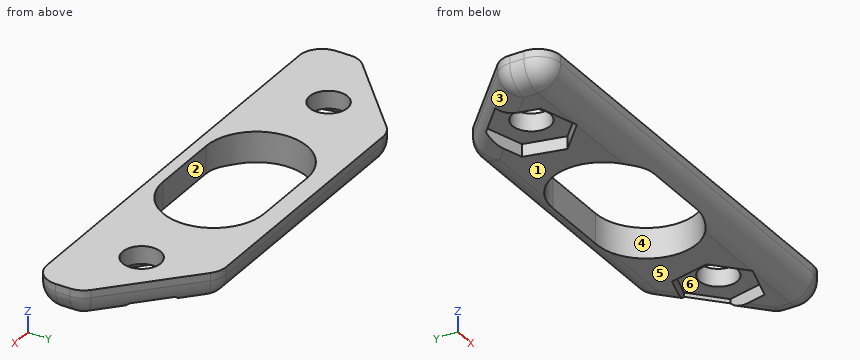
from build123d import *

# Parameters (mm, degrees)
F0_R         = 1.5
F1_DEPTH     = 2.4
F2_DEPTH     = 1
F3_T1_DEPTH  = 1.1190522621
F3_T3_DEPTH  = 32.4
F3_T5_DEPTH  = 20.138628613
F3_T7_DEPTH  = 2.365520331
F3_T9_DEPTH  = 8.3614446785
F3_T11_DEPTH = 8.3614446785
F3_T13_DEPTH = 5.1
F3_T15_DEPTH = 2.5639483811
F3_T20_DEPTH = 1.8
F3_S25_W     = 1.8
F3_S25_H     = 1.8
F3_T26_DEPTH = 1.8
F3_S31_W     = 1.8
F3_S31_H     = 1.8
F3_T32_DEPTH = 1.8
F3_T38_DEPTH = 1.8
F3_T44_DEPTH = 1.8
F3_T50_DEPTH = 1.8


# Not quite as in the source:
# - a fillet or chamfer that OpenCascade refuses, or shapes differently, is made with other operations: its cross-section is extruded or revolved along the edge and cut away or added


with BuildPart() as f1:
    # F0 (on Top) → F1 (new body)
    with BuildSketch(Plane.XY):
        Polygon((-18, -1.2002319389), (-18, -4.9048635534), (18, -4.9048635534), (18, -1.2002319389), (10.7755224389, 5.5), (-10.7755224389, 5.5), align=None)
        Polygon((-9.6294171928, 2.1985610038), (-8.9106989153, -0.9537044309), (-11.2812817225, -3.1522654347), (-14.3705828072, -2.1985610038), (-15.0893010847, 0.9537044309), (-12.7187182775, 3.1522654347), align=None, mode=Mode.SUBTRACT)
        with BuildLine():
            ThreePointArc((-2.75, -4), (-6.75, 0), (-2.75, 4))
            Line((-2.75, 4), (2.75, 4))
            ThreePointArc((2.75, 4), (6.75, 0), (2.75, -4))
            Line((2.75, -4), (-2.75, -4))
        make_face(mode=Mode.SUBTRACT)
        Polygon((9.6294171928, 2.1985610038), (12.7187182775, 3.1522654347), (15.0893010847, 0.9537044309), (14.3705828072, -2.1985610038), (11.2812817225, -3.1522654347), (8.9106989153, -0.9537044309), align=None, mode=Mode.SUBTRACT)
        Polygon((-11.2812817225, -3.1522654347), (-8.9106989153, -0.9537044309), (-9.6294171928, 2.1985610038), (-12.7187182775, 3.1522654347), (-15.0893010847, 0.9537044309), (-14.3705828072, -2.1985610038), align=None)
        with Locations((-12, 0)):
            Circle(F0_R, mode=Mode.SUBTRACT)
        Polygon((15.0893010847, 0.9537044309), (12.7187182775, 3.1522654347), (9.6294171928, 2.1985610038), (8.9106989153, -0.9537044309), (11.2812817225, -3.1522654347), (14.3705828072, -2.1985610038), align=None)
        with Locations((12, 0)):
            Circle(F0_R, mode=Mode.SUBTRACT)
    extrude(amount=F1_DEPTH)

    # F0 (on Top) → F2 (cut)
    with BuildSketch(Plane.XY):
        Polygon((15.0893010847, 0.9537044309), (12.7187182775, 3.1522654347), (9.6294171928, 2.1985610038), (8.9106989153, -0.9537044309), (11.2812817225, -3.1522654347), (14.3705828072, -2.1985610038), align=None)
        with Locations((12, 0)):
            Circle(F0_R, mode=Mode.SUBTRACT)
        Polygon((-11.2812817225, -3.1522654347), (-8.9106989153, -0.9537044309), (-9.6294171928, 2.1985610038), (-12.7187182775, 3.1522654347), (-15.0893010847, 0.9537044309), (-14.3705828072, -2.1985610038), align=None)
        with Locations((-12, 0)):
            Circle(F0_R, mode=Mode.SUBTRACT)
    extrude(amount=F2_DEPTH, mode=Mode.SUBTRACT)

    # F3: fillet of radius 1.8 on 12 edges, made by hand

    # F3_s2 → F3_t1 (cut)
    with BuildSketch(Plane.XZ.offset(1.9858112913)):
        with BuildLine():
            ThreePointArc((-18, 1.8), (-17.4727922061, 0.5272077939), (-16.2, 0))
            Line((-16.2, 0), (-18, 0))
            Line((-18, 0), (-18, 1.8))
        make_face()
        with BuildLine():
            ThreePointArc((16.2, 0), (17.4727922061, 0.5272077939), (18, 1.8))
            Line((18, 1.8), (18, 0))
            Line((18, 0), (16.2, 0))
        make_face()
    extrude(amount=F3_T1_DEPTH, mode=Mode.SUBTRACT)

    # F3_s4 → F3_t3 (cut)
    with BuildSketch(Plane.YZ.offset(-16.2)):
        with BuildLine():
            ThreePointArc((-4.9048635534, 1.8), (-4.3776557595, 0.5272077939), (-3.1048635534, 0))
            Line((-3.1048635534, 0), (-4.9048635534, 0))
            Line((-4.9048635534, 0), (-4.9048635534, 1.8))
        make_face()
    extrude(amount=F3_T3_DEPTH, mode=Mode.SUBTRACT)

    # F3_s6 → F3_t5 (cut)
    with BuildSketch(Plane.YZ.offset(-10.0693143065)):
        with BuildLine():
            ThreePointArc((3.7, 0), (4.9727922061, 0.5272077939), (5.5, 1.8))
            Line((5.5, 1.8), (5.5, 0))
            Line((5.5, 0), (3.7, 0))
        make_face()
    extrude(amount=F3_T5_DEPTH, mode=Mode.SUBTRACT)

    # F3_s8 → F3_t7 (cut)
    with BuildSketch(Plane.XY.offset(1.8)):
        with BuildLine():
            ThreePointArc((10.0693143065, 5.5), (10.7267347006, 5.3756486581), (11.2933205301, 5.0197760282))
            Line((11.2933205301, 5.0197760282), (10.7755224389, 5.5))
            Line((10.7755224389, 5.5), (10.0693143065, 5.5))
        make_face()
        with BuildLine():
            ThreePointArc((-11.2933205301, 5.0197760282), (-10.7267347006, 5.3756486581), (-10.0693143065, 5.5))
            Line((-10.0693143065, 5.5), (-10.7755224389, 5.5))
            Line((-10.7755224389, 5.5), (-11.2933205301, 5.0197760282))
        make_face()
    extrude(amount=F3_T7_DEPTH, mode=Mode.SUBTRACT)

    # F3_s10 → F3_t9 (cut)
    with BuildSketch(Plane(origin=(-3.5684530391, -3.3095075488, 0), x_dir=(0, 0, 1), z_dir=(-0.7332089046, -0.6800034575, 0))):
        with BuildLine():
            ThreePointArc((1.8, 11.3600414903), (0.5272077939, 10.8328336964), (0, 9.5600414903))
            Line((0, 9.5600414903), (0, 11.3600414903))
            Line((0, 11.3600414903), (1.8, 11.3600414903))
        make_face()
    extrude(amount=F3_T9_DEPTH, mode=Mode.SUBTRACT)

    # F3_s12 → F3_t11 (cut)
    with BuildSketch(Plane(origin=(9.6991387326, -8.9953188401, 0), x_dir=(0, 0, 1), z_dir=(-0.7332089046, 0.6800034575, 0))):
        with BuildLine():
            ThreePointArc((0, 9.5600414903), (0.5272077939, 10.8328336964), (1.8, 11.3600414903))
            Line((1.8, 11.3600414903), (0, 11.3600414903))
            Line((0, 11.3600414903), (0, 9.5600414903))
        make_face()
    extrude(amount=F3_T11_DEPTH, mode=Mode.SUBTRACT)

    # F3_s14 → F3_t13 (cut)
    with BuildSketch(Plane.XY.offset(1.8)):
        with BuildLine():
            ThreePointArc((-18, -3.1048635534), (-17.4727922061, -4.3776557595), (-16.2, -4.9048635534))
            Line((-16.2, -4.9048635534), (-18, -4.9048635534))
            Line((-18, -4.9048635534), (-18, -3.1048635534))
        make_face()
        with BuildLine():
            ThreePointArc((16.2, -4.9048635534), (17.4727922061, -4.3776557595), (18, -3.1048635534))
            Line((18, -3.1048635534), (18, -4.9048635534))
            Line((18, -4.9048635534), (16.2, -4.9048635534))
        make_face()
    extrude(amount=F3_T13_DEPTH, mode=Mode.SUBTRACT)

    # F3_s16 → F3_t15 (cut)
    with BuildSketch(Plane.XY.offset(1.8)):
        with BuildLine():
            ThreePointArc((-18, -1.9858112913), (-17.8497289478, -1.265815181), (-17.4240062235, -0.666035263))
            Line((-17.4240062235, -0.666035263), (-18, -1.2002319389))
            Line((-18, -1.2002319389), (-18, -1.9858112913))
        make_face()
        with BuildLine():
            ThreePointArc((18, -1.9858112913), (17.8497289478, -1.265815181), (17.4240062235, -0.666035263))
            Line((17.4240062235, -0.666035263), (18, -1.2002319389))
            Line((18, -1.2002319389), (18, -1.9858112913))
        make_face()
    extrude(amount=F3_T15_DEPTH, mode=Mode.SUBTRACT)


with BuildPart() as f3_tool18:
    # F3_s19 → F3_t20 (new body)
    with BuildSketch(Plane.XY.offset(1.8)):
        Polygon((-16.2, -1.9858112913), (-18, -1.9858112913), (-18, -1.2002319389), (-17.4240062235, -0.666035263), align=None)
    extrude(amount=-F3_T20_DEPTH)

    # F3_s21 → F3_t22 (revolve, cut)
    with BuildSketch(Plane(origin=(-16.2, -1.9858112913, 1.8), x_dir=(0.9165160821, -0.399997839, 0), z_dir=(0.399997839, 0.9165160821, 0))):
        with BuildLine():
            ThreePointArc((0, -1.8), (1.8, 0), (0, 1.8))
            Line((0, 1.8), (0, -1.8))
        make_face()
    revolve(axis=Axis((-16.2, -1.9858112913, 1.8), (0, 0, -1)), mode=Mode.SUBTRACT)


with BuildPart() as f1_1:
    add(f1.part)

    # F3_t17: cut F3_tool18
    add(f3_tool18.part, mode=Mode.SUBTRACT)


with BuildPart() as f3_tool24:
    # F3_s25 → F3_t26 (new body)
    with BuildSketch(Plane.YZ.offset(-16.2)):
        with Locations((-4.0048635534, 0.9)):
            Rectangle(F3_S25_W, F3_S25_H)
    extrude(amount=-F3_T26_DEPTH)

    # F3_s27 → F3_t28 (revolve, cut)
    with BuildSketch(Plane(origin=(-16.2, -3.1048635534, 1.8), x_dir=(0, 0.7071067812, 0.7071067812), z_dir=(0, -0.7071067812, 0.7071067812))):
        with BuildLine():
            ThreePointArc((0, -1.8), (1.8, 0), (0, 1.8))
            Line((0, 1.8), (0, -1.8))
        make_face()
    revolve(axis=Axis((-16.2, -3.1048635534, 1.8), (-1, 0, 0)), mode=Mode.SUBTRACT)


with BuildPart() as f1_2:
    add(f1_1.part)

    # F3_t23: cut F3_tool24
    add(f3_tool24.part, mode=Mode.SUBTRACT)


with BuildPart() as f3_tool30:
    # F3_s31 → F3_t32 (new body)
    with BuildSketch(Plane.XZ.offset(3.1048635534)):
        with Locations((17.1, 0.9)):
            Rectangle(F3_S31_W, F3_S31_H)
    extrude(amount=F3_T32_DEPTH)

    # F3_s33 → F3_t34 (revolve, cut)
    with BuildSketch(Plane(origin=(16.2, -3.1048635534, 1.8), x_dir=(-0.7071067812, 0, 0.7071067812), z_dir=(0.7071067812, 0, 0.7071067812))):
        with BuildLine():
            ThreePointArc((0, -1.8), (1.8, 0), (0, 1.8))
            Line((0, 1.8), (0, -1.8))
        make_face()
    revolve(axis=Axis((16.2, -3.1048635534, 1.8), (0, -1, 0)), mode=Mode.SUBTRACT)


with BuildPart() as f1_3:
    add(f1_2.part)

    # F3_t29: cut F3_tool30
    add(f3_tool30.part, mode=Mode.SUBTRACT)


with BuildPart() as f3_tool36:
    # F3_s37 → F3_t38 (new body)
    with BuildSketch(Plane.XY.offset(1.8)):
        Polygon((16.2, -1.9858112913), (18, -1.9858112913), (18, -1.2002319389), (17.4240062235, -0.666035263), align=None)
    extrude(amount=-F3_T38_DEPTH)

    # F3_s39 → F3_t40 (revolve, cut)
    with BuildSketch(Plane(origin=(16.2, -1.9858112913, 1.8), x_dir=(-0.9165160821, -0.399997839, 0), z_dir=(0.399997839, -0.9165160821, 0))):
        with BuildLine():
            ThreePointArc((0, -1.8), (1.8, 0), (0, 1.8))
            Line((0, 1.8), (0, -1.8))
        make_face()
    revolve(axis=Axis((16.2, -1.9858112913, 1.8), (0, 0, -1)), mode=Mode.SUBTRACT)


with BuildPart() as f1_4:
    add(f1_3.part)

    # F3_t35: cut F3_tool36
    add(f3_tool36.part, mode=Mode.SUBTRACT)


with BuildPart() as f3_tool42:
    # F3_s43 → F3_t44 (new body)
    with BuildSketch(Plane.XY.offset(1.8)):
        Polygon((10.0693143065, 3.7), (10.0693143065, 5.5), (10.7755224389, 5.5), (11.2933205301, 5.0197760282), align=None)
    extrude(amount=-F3_T44_DEPTH)

    # F3_s45 → F3_t46 (revolve, cut)
    with BuildSketch(Plane(origin=(10.0693143065, 3.7, 1.8), x_dir=(-0.3652335523, -0.9309159212, 0), z_dir=(0.9309159212, -0.3652335523, 0))):
        with BuildLine():
            ThreePointArc((0, -1.8), (1.8, 0), (0, 1.8))
            Line((0, 1.8), (0, -1.8))
        make_face()
    revolve(axis=Axis((10.0693143065, 3.7, 1.8), (0, 0, -1)), mode=Mode.SUBTRACT)


with BuildPart() as f1_5:
    add(f1_4.part)

    # F3_t41: cut F3_tool42
    add(f3_tool42.part, mode=Mode.SUBTRACT)


with BuildPart() as f3_tool48:
    # F3_s49 → F3_t50 (new body)
    with BuildSketch(Plane.XY.offset(1.8)):
        Polygon((-10.0693143065, 3.7), (-10.0693143065, 5.5), (-10.7755224389, 5.5), (-11.2933205301, 5.0197760282), align=None)
    extrude(amount=-F3_T50_DEPTH)

    # F3_s51 → F3_t52 (revolve, cut)
    with BuildSketch(Plane(origin=(-10.0693143065, 3.7, 1.8), x_dir=(0.3652335523, -0.9309159212, 0), z_dir=(0.9309159212, 0.3652335523, 0))):
        with BuildLine():
            ThreePointArc((0, -1.8), (1.8, 0), (0, 1.8))
            Line((0, 1.8), (0, -1.8))
        make_face()
    revolve(axis=Axis((-10.0693143065, 3.7, 1.8), (0, 0, -1)), mode=Mode.SUBTRACT)


with BuildPart() as f1_6:
    add(f1_5.part)

    # F3_t47: cut F3_tool48
    add(f3_tool48.part, mode=Mode.SUBTRACT)


solid = f1_6.part
Model file for the job. Use its own axes, mm. Face numbers are marked on the shaded views. A direction names the side the tool comes from. Coordinates: 2 decimals unless noted, no trailing zeros. Write each loop counter-clockwise with the first axis right and the second up, starting at its lowest first coordinate (ties: lowest second). Pieces come first, ordered by that corner, then holes. Notation, with made-up numbers: (-28.5, 25) - (-22.5, 25) arc R22 ccw to (-22.5, 49) - close; hole circle Ø3 at (9.25, 41). An arc over 180 degrees is marked (long way). Write each question's results on one line, items separated by ' | '. Start each with the question number.
1) Flat gauge pins, fed straight in: P1, Ø1, axis at x = 2.5, y = -2, coming from the -Z side; P2, Ø3.5, axis at x = 12, y = 0, coming from the -Z side; P3, Ø1.2, axis at x = -1, z = 1, coming from the -Y side. Where does each tip first touch, or does it go through?
2) Mould opens along X. For the marked faces 1, 2 and 3 say: pulls with the +X half, pulls with the -X half, needs draft (parallel to the pull), parting line crosses it, or undercut.
3) Probe line 1 along X through (y, z) = (-0.75, 1.9); line 2 along Z through (x, y) = (10, -4); line 3 along Y through (x, z) = (-12, 1.85). List the from-to ranges inside material, lowest first. Write a range as from..to.
4) Cut at A-A (x = 0). Write the cut outline in (y, z), then the cut area to 3 significant figures.
5) Cut at B-B (y = 0). Count the separate pieces of the cut face and the enclosed holes in it, then the cut area to 3 significant figures.
6) Cut at C-C (x = -8.5). Write the cut outline in (y, z).
7) 3-axis set-ups, long thin cutter, end or side, ignore diameter. For the marked faces 4, 5 and 6: which of +Z, -Z, +X, -X, +Y, -Y reach the whole face in a straight line?
Returned:
1) P1: through | P2: z = 1 | P3: y = -4.89
2) face 1: needs draft | face 2: undercut | face 3: pulls with the -X half
3) line 1: -17.51..-13.3, -10.7..-6.68, 6.68..10.7, 13.3..17.51 | line 2: 0.24..2.4 | line 3: -4.9..-1.5, 1.5..4.36
4) outline: (-4.9, 1.8) arc R1.8 ccw to (-4, 0.24) - (-4, 2.4) - (-4.9, 2.4) - close; (4, 0.03) arc R1.8 ccw to (5.5, 1.8) - (5.5, 2.4) - (4, 2.4) - close | area: 4.45 mm^2
5) separate pieces: 4 | enclosed holes: 0 | area: 25.9 mm^2
6) outline: (-4.9, 1.8) arc R1.8 ccw to (-3.1, 0) - (3.7, 0) arc R1.8 ccw to (5.5, 1.8) - (5.5, 2.4) - (-4.9, 2.4) - close
7) face 4: +Z, -Z | face 5: -Z, +X, -X, +Y, -Y | face 6: -Z
